```python
from build123d import *

# Parameters (mm, degrees)
BOSS_EXTRUDE1_DEPTH = 1.6
CUT_EXTRUDE1_DEPTH  = 1.6
SKETCH5_R           = 1.5
CUT_EXTRUDE2_DEPTH  = 1.6
BOSS_EXTRUDE2_DEPTH = 1.6
SKETCH10_R          = 1.5
CUT_EXTRUDE5_DEPTH  = 1.6
CUT_EXTRUDE6_DEPTH  = 1.6
SKETCH14_W          = 40
SKETCH14_H          = 25
CUT_EXTRUDE7_DEPTH  = 1.6
CUT_EXTRUDE10_DEPTH = 1.6


with BuildPart() as part:
    # Sketch3 → Boss-Extrude1 (new body)
    with BuildSketch(Plane(origin=(0, 0, 0), x_dir=(1, 0, 0), z_dir=(0, 1, 0))):
        Polygon((-20, 65), (20, 65), (65, 39.019237886), (65, -39.019237886), (20, -65), (-20, -65), (-65, -39.019237886), (-65, 39.019237886), align=None)
    extrude(amount=BOSS_EXTRUDE1_DEPTH)

    # Sketch4 → Cut-Extrude1 (cut)
    with BuildSketch(Plane(origin=(0, 1.6, 0), x_dir=(1, 0, 0), z_dir=(0, 1, 0))):
        Polygon((-61.579798567, 40.993892105), (-65, 31.596965897), (-65, 39.019237886), align=None)
        Polygon((65, 31.596965897), (61.579798567, 40.993892105), (65, 39.019237886), align=None)
        Polygon((61.579798567, -40.993892105), (65, -39.019237886), (65, -31.596965897), align=None)
        Polygon((-61.579798567, -40.993892105), (-65, -39.019237886), (-65, -31.596965897), align=None)
    extrude(amount=-CUT_EXTRUDE1_DEPTH, mode=Mode.SUBTRACT)

    # Sketch5 → Cut-Extrude2 (cut)
    with BuildSketch(Plane(origin=(0, 1.6, 0), x_dir=(1, 0, 0), z_dir=(0, 1, 0))):
        with Locations(Location((-30, 50, 0), (0, 0, 270))):
            Circle(SKETCH5_R)
        with Locations(Location((30, 50, 0), (0, 0, 270))):
            Circle(SKETCH5_R)
        with Locations(Location((30, -50, 0), (0, 0, 270))):
            Circle(SKETCH5_R)
        with Locations(Location((-30, -50, 0), (0, 0, 270))):
            Circle(SKETCH5_R)
    extrude(amount=-CUT_EXTRUDE2_DEPTH, mode=Mode.SUBTRACT)

    # Sketch6 → Boss-Extrude2 (add)
    with BuildSketch(Plane(origin=(0, 1.6, 0), x_dir=(1, 0, 0), z_dir=(0, 1, 0))):
        Polygon((-65, 31.596965897), (-76.50035508, 0), (-65, -31.596965897), align=None)
        Polygon((65, 31.596965897), (65, -31.596965897), (76.50035508, 0), align=None)
    extrude(amount=-BOSS_EXTRUDE2_DEPTH)

    # Sketch10 → Cut-Extrude5 (cut)
    with BuildSketch(Plane(origin=(0, 1.6, 0), x_dir=(1, 0, 0), z_dir=(0, 1, 0))):
        with Locations(Location((-28.953010595, 34.50485439, 0), (0, 0, 270))):
            Circle(SKETCH10_R)
        with Locations(Location((28.953010595, 34.50485439, 0), (0, 0, 270))):
            Circle(SKETCH10_R)
        with Locations(Location((-28.953010595, -34.50485439, 0), (0, 0, 270))):
            Circle(SKETCH10_R)
        with Locations(Location((28.953010595, -34.50485439, 0), (0, 0, 270))):
            Circle(SKETCH10_R)
    extrude(amount=-CUT_EXTRUDE5_DEPTH, mode=Mode.SUBTRACT)

    # Sketch11 → Cut-Extrude6 (cut)
    with BuildSketch(Plane(origin=(0, 1.6, 0), x_dir=(1, 0, 0), z_dir=(0, 1, 0))):
        Polygon((-68.311024809, 22.5), (-68.311024809, -22.5), (-76.50035508, 0), align=None)
        Polygon((68.311024809, 22.5), (68.311024809, -22.5), (76.50035508, 0), align=None)
    extrude(amount=-CUT_EXTRUDE6_DEPTH, mode=Mode.SUBTRACT)

    # Sketch14 → Cut-Extrude7 (cut)
    with BuildSketch(Plane(origin=(0, 1.6, 0), x_dir=(1, 0, 0), z_dir=(0, 1, 0))):
        with Locations((0, 52.5)):
            Rectangle(SKETCH14_W, SKETCH14_H)
    extrude(amount=-CUT_EXTRUDE7_DEPTH, mode=Mode.SUBTRACT)

    # Sketch17 → Cut-Extrude10 (cut)
    with BuildSketch(Plane(origin=(0, 1.6, 0), x_dir=(1, 0, 0), z_dir=(0, 1, 0))):
        Polygon((-56.311024809, 44.035820052), (-56.311024809, -44.035820052), (-61.579798567, -40.993892105), (-68.311024809, -22.5), (-68.311024809, 22.5), (-61.579798567, 40.993892105), align=None)
        Polygon((68.311024809, 22.5), (61.579798567, 40.993892105), (56.311024809, 44.035820052), (56.311024809, -44.035820052), (61.579798567, -40.993892105), (68.311024809, -22.5), align=None)
    extrude(amount=-CUT_EXTRUDE10_DEPTH, mode=Mode.SUBTRACT)


solid = part.part
```
Read the model definition and answer for the solid it produces. Units are mm, in the model's axes. Give positions to 0.01 mm unless a question says otherwise; leave off trailing zeros. Order: outer loops, then holes, each group sorted by start corner. A loop starts at its lowest first (then second) coordinate and runs counter-clockwise, first axis right, second up. Notation, with made-up numbers: (20, 40) -> (63, 40) arc R25 ccw to (63, 65) -> close; hole circle Ø10 at (18.25, 28.25). An arc over 180 degrees is marked (long way). One line per item, written item: value. Start each with the question number.
(1) The part is cut by section A-A (z = -50). Determine the outline of the cut face in (x, y), and give its area (3 significant figures).
(2) Flat-ended cylindrical pins translate along their axes: P1, Ø0.5, axis at y = 0.5, z = -53, coming from the -X side; P2, Ø0.5, axis at x = 7, y = 0.5, coming from the -Z side. Find the tip coordinate at first contact, or state that the pin passes through.
(3) The part is cut by section B-B (y = 1). State how many separate pieces and enclosed holes the cut face has, and give its area (3 significant figures).
(4) Straight lines are drawn through the part: L1, parallel to X at y = 0.9, z = 50; L2, parallel to X at y = 1, z = 33.5; L3, parallel to X at y = 1.15, z = -50. For each, find the intervals that lie inside material, in ascending order.
(5) The part is cut by section D-D (x = -17). Determine the outline of the cut face in (y, z).
(6) For a pull along Z with two mould halves and no side action, classify faces 1 (the flat face through (37.901, 0.789, -54.665)), 2 (the cylindrical face through (-28.99, 0.81, 48.89)), 3 (the flat face through (-1, 1.6, -1)) as released by +Z, released by -Z, zero draft, split by the parting line, or undercut.
(7) The part is cut by section C-C (z = 50). Determine the outline of the cut face in (x, y).
Taken from the geometry:
1. outline: (-45.98, 0) -> (-31.5, 0) -> (-31.5, 1.6) -> (-45.98, 1.6) -> close; (-28.5, 0) -> (-20, 0) -> (-20, 1.6) -> (-28.5, 1.6) -> close; (20, 0) -> (28.5, 0) -> (28.5, 1.6) -> (20, 1.6) -> close; (31.5, 0) -> (45.98, 0) -> (45.98, 1.6) -> (31.5, 1.6) -> close
1. area: 73.5 mm^2
2. P1: x = -41.22
2. P2: z = -40
3. separate pieces: 1
3. enclosed holes: 8
3. area: 12,100 mm^2
4. L1: -45.98 to -31.5, -28.5 to 28.5, 31.5 to 45.98
4. L2: -56.31 to -30.07, -27.84 to 27.84, 30.07 to 56.31
4. L3: -45.98 to -31.5, -28.5 to -20, 20 to 28.5, 31.5 to 45.98
5. outline: (0, -40) -> (1.6, -40) -> (1.6, 65) -> (0, 65) -> close
6. face 1: released by -Z
6. face 2: undercut
6. face 3: zero draft
7. outline: (-45.98, 0) -> (-31.5, 0) -> (-31.5, 1.6) -> (-45.98, 1.6) -> close; (-28.5, 0) -> (28.5, 0) -> (28.5, 1.6) -> (-28.5, 1.6) -> close; (31.5, 0) -> (45.98, 0) -> (45.98, 1.6) -> (31.5, 1.6) -> close
